```python
from build123d import *

# Parameters (mm, degrees)
F1_DEPTH  = 16.002
F2_R      = 9.652
F3_W      = 76.2
F3_H      = 29.972
F4_DEPTH  = 16.002
F5_R      = 14.224
F6_R      = 9.652
F7_R      = 6.35
F8_DEPTH  = 16.003
F10_DEPTH = 16.003


with BuildPart() as f1:
    # F0 (on Front) → F1 (new body)
    with BuildSketch(Plane.XZ):
        with BuildLine():
            Line((0, 44.45), (0, 0))
            Line((0, 0), (101.6, 0))
            Line((101.6, 0), (101.6, 44.45))
            ThreePointArc((101.6, 44.45), (88.9, 57.15), (76.2, 44.45))
            Line((76.2, 44.45), (76.2, 16.002))
            Line((76.2, 16.002), (25.4, 16.002))
            Line((25.4, 16.002), (25.4, 44.45))
            ThreePointArc((25.4, 44.45), (12.7, 57.15), (0, 44.45))
        make_face()
    extrude(amount=F1_DEPTH)

    # F2
    f2_edges = [f1.edges().sort_by_distance(p)[0] for p in [
        (25.4, -8.001, 16.002),
        (76.2, -8.001, 16.002),
    ]]
    fillet(f2_edges, radius=F2_R)

    # F3 (on Top) → F4 (join)
    with BuildSketch(Plane.XY):
        with Locations((50.8, -30.988)):
            Rectangle(F3_W, F3_H)
    extrude(amount=F4_DEPTH)

    # F5
    f5_edges = [f1.edges().sort_by_distance(p)[0] for p in [
        (88.9, -45.974, 8.001),
        (12.7, -45.974, 8.001),
    ]]
    fillet(f5_edges, radius=F5_R)

    # F6
    f6_edges = [f1.edges().sort_by_distance(p)[0] for p in [
        (88.9, -16.002, 8.001),
        (12.7, -16.002, 8.001),
    ]]
    fillet(f6_edges, radius=F6_R)

    # F7 (on face) → F8 (cut, through all)
    with BuildSketch(Plane.XZ.offset(16.002)):
        with Locations((12.7, 44.45)):
            Circle(F7_R)
        with Locations((88.9, 44.45)):
            Circle(F7_R)
    extrude(amount=-F8_DEPTH, mode=Mode.SUBTRACT)

    # F9 (on face) → F10 (cut, through all)
    with BuildSketch(Plane.XY.offset(16.002)):
        with BuildLine():
            Line((69.85, -25.4), (31.75, -25.4))
            ThreePointArc((31.75, -25.4), (25.4, -31.75), (31.75, -38.1))
            Line((31.75, -38.1), (69.85, -38.1))
            ThreePointArc((69.85, -38.1), (76.2, -31.75), (69.85, -25.4))
        make_face()
    extrude(amount=-F10_DEPTH, mode=Mode.SUBTRACT)


solid = f1.part
```
CAD build for the part. Positions are in the model's coordinates, mm. A direction names the side the tool comes from. Give positions to 0.01 mm unless a question says otherwise; leave off trailing zeros. Order: outer loops, then holes, each group sorted by start corner. A loop starts at its lowest first (then second) coordinate and runs counter-clockwise, first axis right, second up. Notation, with made-up numbers: M -24.5,-4.75 L -19.5,-4.75 A22 ccw -19.5,28.25 Z; hole C -14.5,42.5 d3. An arc over 180 degrees is marked long. Put each result on its own line as item: value. Start each with the question number.
(1) Saw through at A-A, the plane y = -4. Write the cut outline in (x, z).
(2) Which spindle directions (+Z, -Z, +X, -X, +Y, -Y) get a long thin tool onto all of the face, cutting with end or side? Do faces 4 (the cylindrical face through (73.448, -8.113, 18.904)), 5 (the flat face through (50, -23, 16.002)), 6 (the flat face through (88.9, -29, 8)), 7 (the flat face through (51, -38.1, 8)), 8 (the flat face through (50, 0, 10)). Say none if no direction does.
(3) Saw through at D-D, the plane z = 9.5. Write the cut outline in (x, y), then the cut area to 3 significant figures.
(4) Saw through at B-B, the plane z = 49. Write the cut outline in (x, y), then the cut area to 3 significant figures.
(5) Mould opens along X. For faces 1 (the cylindrical face through (11.873, -8.113, 50.746)), 2 (the cylindrical face through (84.62, -41.92, 8.11)), 3 (the flat face through (13, -16.002, 29)) say: +X half, -X half, draft (parallel to the pull), parting line (faces both ways), or undercut.
(6) Drill centre lines: line 1 along X through (y, z) = (-6, 44); line 2 along X through (y, z) = (-5.5, 27.5); line 3 along Y through (x, z) = (40, 7). Where is each one in solid material? Low to high.
(7) Saw through at C-C, the plane x = 33. Write the cut outline in (y, z), then the cut area to 3 significant figures.
(8) Flat gauge pins, fed straight in: pin 1 Ø4 at (x, z) = (11, 20) entering from -Y; pin 2 Ø1.8 at (y, z) = (-29.5, 6.5) entering from -X; pin 3 Ø1.5 at (y, z) = (-12, 51) entering from +X; pin 4 Ø1 at (x, z) = (54, 18) entering from -Y. Where does each tip first touch, or does it go through?
Check result:
1. outline: M 0,0 L 101.6,0 L 101.6,44.45 A12.7 ccw 76.2,44.45 L 76.2,25.65 A9.65 cw 66.55,16 L 35.05,16 A9.65 cw 25.4,25.65 L 25.4,44.45 A12.7 ccw 0,44.45 Z; hole C 12.7,44.45 d12.7; hole C 88.9,44.45 d12.7
2. face 4: +Z, +Y, -Y
2. face 5: +Z, -Y
2. face 6: +Z, -Z, +X, -Y
2. face 7: +Z, -Z
2. face 8: +Z, -Z, +X, -X, +Y
3. outline: M 0,-16 L 3.05,-16 A9.65 cw 12.7,-25.65 L 12.7,-31.75 A14.22 ccw 26.92,-45.97 L 74.68,-45.97 A14.22 ccw 88.9,-31.75 L 88.9,-25.65 A9.65 cw 98.55,-16 L 101.6,-16 L 101.6,0 L 0,0 Z; hole M 31.75,-38.1 L 69.85,-38.1 A6.35 ccw 69.85,-25.4 L 31.75,-25.4 A6.35 ccw Z
3. area: 3,250 mm2
4. outline: M 0.84,-16 L 8.27,-16 L 8.27,0 L 0.84,0 Z; M 17.13,-16 L 24.56,-16 L 24.56,0 L 17.13,0 Z; M 77.04,-16 L 84.47,-16 L 84.47,0 L 77.04,0 Z; M 93.33,-16 L 100.76,-16 L 100.76,0 L 93.33,0 Z
4. area: 475 mm2
5. face 1: undercut
5. face 2: +X half
5. face 3: draft
6. line 1: x = 0 to 6.37, 19.03 to 25.4, 76.2 to 82.57, 95.23 to 101.6
6. line 2: x = 0 to 25.4, 76.2 to 101.6
6. line 3: y = -45.97 to -38.1, -25.4 to 0
7. outline: M -45.97,0 L -38.1,0 L -38.1,16 L -45.97,16 Z; M -25.4,0 L 0,0 L 0,16.22 L -16,16.22 L -16,16 L -25.4,16 Z
7. area: 536 mm2
8. pin 1: stops at y = -16
8. pin 2: stops at x = 12.7
8. pin 3: stops at x = 100.2
8. pin 4: passes through
